Verification items for the finished model (mm, model axes). Face numbers are marked on the shaded views. A direction names the side the tool comes from. Coordinates: 2 decimals unless noted, no trailing zeros. Write each loop counter-clockwise with the first axis right and the second up, starting at its lowest first coordinate (ties: lowest second). Pieces come first, ordered by that corner, then holes. Notation, with made-up numbers: M 54.5,58.5 L 88.5,58.5 A6 ccw 88.5,67.5 Z; hole C 6,-30 d11. An arc over 180 degrees is marked long. Answer in a Markdown table with one row per item.
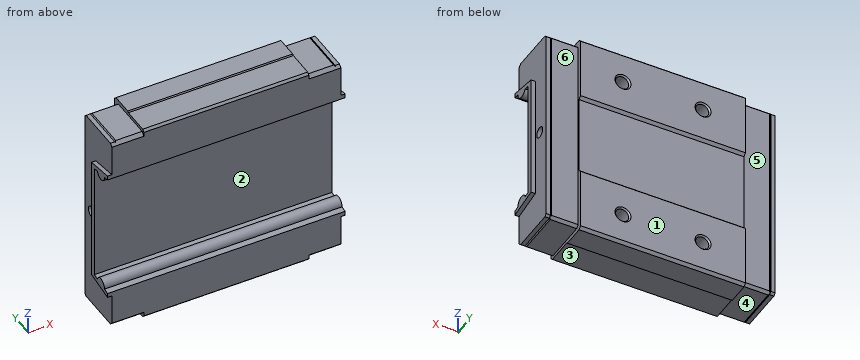
from build123d import *

# Parameters (mm, degrees)
RESSALTO_EXTRUS_O1_DEPTH      = 15.45
RESSALTO_EXTRUS_O1_DEPTH_BACK = 15.45
RESSALTO_EXTRUS_O2_DEPTH      = 6
RESSALTO_EXTRUS_O3_DEPTH      = 6
RESSALTO_EXTRUS_O4_DEPTH      = 22.25
RESSALTO_EXTRUS_O4_DEPTH_BACK = 22.25
CORTE_EXTRUS_O1_DEPTH         = 22.25
CORTE_EXTRUS_O1_DEPTH_BACK    = 22.25
ESBO_O10_W                    = 48.5
ESBO_O10_H                    = 44
CORTE_EXTRUS_O2_DEPTH         = 11
CORTE_EXTRUS_O3_DEPTH         = 20
CORTE_EXTRUS_O3_DEPTH_BACK    = 20
CORTE_EXTRUS_O4_DEPTH         = 20
CORTE_EXTRUS_O4_DEPTH_BACK    = 20
CORTE_EXTRUS_O5_DEPTH         = 10
CORTE_EXTRUS_O6_DEPTH         = 10
CORTE_EXTRUS_O7_DEPTH         = 10
CORTE_EXTRUS_O8_DEPTH         = 10
ESBO_O17_W                    = 2.5
ESBO_O17_H                    = 1
ESBO_O18_W                    = 2.5
ESBO_O18_H                    = 1


with BuildPart() as part:
    # Esboço1 → Ressalto-extrusão1 (new, two sides: drawn at the far end of the back side and taken through both)
    with BuildSketch(Plane(origin=(0, 0, 0), x_dir=(0, 0, -1), z_dir=(1, 0, 0)).offset(-RESSALTO_EXTRUS_O1_DEPTH_BACK)):
        Polygon((-20, 9.5), (-20, 5.5), (-19.8, 5.3), (-19.8, 0.4), (-19.4, 0), (19.4, 0), (19.8, 0.4), (19.8, 5.3), (20, 5.5), (20, 9.5), (19.5, 10), (8, 10), (7.5, 9.5), (-7.5, 9.5), (-8, 10), (-19.5, 10), align=None)
    extrude(amount=RESSALTO_EXTRUS_O1_DEPTH + RESSALTO_EXTRUS_O1_DEPTH_BACK)

    # Esboço2 → Ressalto-extrusão2 (add)
    with BuildSketch(Plane(origin=(-15.45, 0, 0), x_dir=(0, 0, -1), z_dir=(1, 0, 0))):
        Polygon((-19.2, 8.7), (-19.2, 0.6), (-18.6, 0), (18.6, 0), (19.2, 0.6), (19.2, 8.7), (18.7, 9.2), (-18.7, 9.2), align=None)
    extrude(amount=-RESSALTO_EXTRUS_O2_DEPTH)

    # Esboço3 → Ressalto-extrusão3 (add)
    with BuildSketch(Plane(origin=(15.45, 0, 0), x_dir=(0, 0, -1), z_dir=(1, 0, 0))):
        Polygon((-19.2, 8.7), (-19.2, 0.6), (-18.6, 0), (18.6, 0), (19.2, 0.6), (19.2, 8.7), (18.7, 9.2), (-18.7, 9.2), align=None)
    extrude(amount=RESSALTO_EXTRUS_O3_DEPTH)

    # Esboço4 → Ressalto-extrusão4 (add, two sides: drawn at the far end of the back side and taken through both)
    with BuildSketch(Plane(origin=(0, 0, 0), x_dir=(0, 0, -1), z_dir=(1, 0, 0)).offset(-RESSALTO_EXTRUS_O4_DEPTH_BACK)):
        Polygon((-12.816, 0), (12.816, 0), (11.846201606, 5.5), (-11.846201606, 5.5), align=None)
    extrude(amount=RESSALTO_EXTRUS_O4_DEPTH + RESSALTO_EXTRUS_O4_DEPTH_BACK)

    # Esboço5 → Corte-extrusão1 (cut, two sides: drawn at the far end of the back side and taken through both)
    with BuildSketch(Plane(origin=(0, 0, 0), x_dir=(0, 0, -1), z_dir=(1, 0, 0)).offset(-CORTE_EXTRUS_O1_DEPTH_BACK)):
        with BuildLine():
            Line((-12, 0), (12, 0))
            Line((12, 0), (11.814562479, 1.051668439))
            ThreePointArc((11.814562479, 1.051668439), (10.518990309, 2.082939778), (11.383714346, 3.495129625))
            Line((11.383714346, 3.495129625), (11.206528587, 4.5))
            Line((11.206528587, 4.5), (-11.206528587, 4.5))
            Line((-11.206528587, 4.5), (-11.383714346, 3.495129625))
            ThreePointArc((-11.383714346, 3.495129625), (-10.518990309, 2.082939778), (-11.814562479, 1.051668439))
            Line((-11.814562479, 1.051668439), (-12, 0))
        make_face()
    extrude(amount=CORTE_EXTRUS_O1_DEPTH + CORTE_EXTRUS_O1_DEPTH_BACK, mode=Mode.SUBTRACT)

    # Esboço6 → Corte-Revolução1 (revolve, cut)
    with BuildSketch(Plane.XY.offset(14), mode=Mode.PRIVATE) as corte_revolu_o1_sk:
        Polygon((7.5, 10), (9, 10), (8.7295, 9.7295), (8.7295, 5.8), (7.5, 5.090147844), align=None)
    revolve(corte_revolu_o1_sk.sketch.rotate(Axis((7.5, 5.090147844, 14), (0, 1, 0)), 270), axis=Axis((7.5, 5.090147844, 14), (0, 1, 0)), mode=Mode.SUBTRACT)

    # Esboço7 → Corte-Revolução2 (revolve, cut)
    with BuildSketch(Plane.XY.offset(-14), mode=Mode.PRIVATE) as corte_revolu_o2_sk:
        Polygon((-7.5, 10), (-6, 10), (-6.2705, 9.7295), (-6.2705, 5.8), (-7.5, 5.090147844), align=None)
    revolve(corte_revolu_o2_sk.sketch.rotate(Axis((-7.5, 5.090147844, -14), (0, 1, 0)), 270), axis=Axis((-7.5, 5.090147844, -14), (0, 1, 0)), mode=Mode.SUBTRACT)

    # Esboço8 → Corte-Revolução3 (revolve, cut)
    with BuildSketch(Plane.XY.offset(14), mode=Mode.PRIVATE) as corte_revolu_o3_sk:
        Polygon((-7.5, 10), (-6, 10), (-6.2705, 9.7295), (-6.2705, 5.8), (-7.5, 5.090147844), align=None)
    revolve(corte_revolu_o3_sk.sketch.rotate(Axis((-7.5, 5.090147844, 14), (0, 1, 0)), 270), axis=Axis((-7.5, 5.090147844, 14), (0, 1, 0)), mode=Mode.SUBTRACT)

    # Esboço9 → Corte-Revolução4 (revolve, cut)
    with BuildSketch(Plane.XY.offset(-14), mode=Mode.PRIVATE) as corte_revolu_o4_sk:
        Polygon((7.5, 10), (9, 10), (8.7295, 9.7295), (8.7295, 5.8), (7.5, 5.090147844), align=None)
    revolve(corte_revolu_o4_sk.sketch.rotate(Axis((7.5, 5.090147844, -14), (0, 1, 0)), 270), axis=Axis((7.5, 5.090147844, -14), (0, 1, 0)), mode=Mode.SUBTRACT)

    # Esboço10 → Corte-extrusão2 (cut)
    with BuildSketch(Plane(origin=(0, 0, 0), x_dir=(1, 0, 0), z_dir=(0, 1, 0))):
        Rectangle(ESBO_O10_W, ESBO_O10_H)
        Polygon((-23.25, 19.1), (-23.25, -19.1), (-20.65, -19.1), (-20.65, -21), (20.65, -21), (20.65, -19.1), (23.25, -19.1), (23.25, 19.1), (20.65, 19.1), (20.65, 21), (-20.65, 21), (-20.65, 19.1), align=None, mode=Mode.SUBTRACT)
    extrude(amount=CORTE_EXTRUS_O2_DEPTH, mode=Mode.SUBTRACT)

    # Esboço11 → Corte-extrusão3 (cut, two sides: drawn at the far end of the back side and taken through both)
    with BuildSketch(Plane.XY.offset(-CORTE_EXTRUS_O3_DEPTH_BACK)):
        Polygon((-20.65, 9.2), (-20.65, 8.95), (-20.4, 9.2), align=None)
    extrude(amount=CORTE_EXTRUS_O3_DEPTH + CORTE_EXTRUS_O3_DEPTH_BACK, mode=Mode.SUBTRACT)

    # Esboço12 → Corte-extrusão4 (cut, two sides: drawn at the far end of the back side and taken through both)
    with BuildSketch(Plane.XY.offset(-CORTE_EXTRUS_O4_DEPTH_BACK)):
        Polygon((20.4, 9.2), (20.65, 8.95), (20.65, 9.2), align=None)
    extrude(amount=CORTE_EXTRUS_O4_DEPTH + CORTE_EXTRUS_O4_DEPTH_BACK, mode=Mode.SUBTRACT)

    # Esboço13 → Corte-extrusão5 (cut)
    with BuildSketch(Plane(origin=(0, 0, 0), x_dir=(1, 0, 0), z_dir=(0, 1, 0))):
        Polygon((-20.65, 19.2), (-20.65, 18.95), (-20.4, 19.2), align=None)
    extrude(amount=CORTE_EXTRUS_O5_DEPTH, mode=Mode.SUBTRACT)

    # Esboço14 → Corte-extrusão6 (cut)
    with BuildSketch(Plane(origin=(0, 0, 0), x_dir=(1, 0, 0), z_dir=(0, 1, 0))):
        Polygon((-20.65, -19.2), (-20.4, -19.2), (-20.65, -18.95), align=None)
    extrude(amount=CORTE_EXTRUS_O6_DEPTH, mode=Mode.SUBTRACT)

    # Esboço15 → Corte-extrusão7 (cut)
    with BuildSketch(Plane(origin=(0, 0, 0), x_dir=(1, 0, 0), z_dir=(0, 1, 0))):
        Polygon((20.4, 19.2), (20.65, 18.95), (20.65, 19.2), align=None)
    extrude(amount=CORTE_EXTRUS_O7_DEPTH, mode=Mode.SUBTRACT)

    # Esboço16 → Corte-extrusão8 (cut)
    with BuildSketch(Plane(origin=(0, 0, 0), x_dir=(1, 0, 0), z_dir=(0, 1, 0))):
        Polygon((20.4, -19.2), (20.65, -19.2), (20.65, -18.95), align=None)
    extrude(amount=CORTE_EXTRUS_O8_DEPTH, mode=Mode.SUBTRACT)

    # Esboço17 → Corte-Revolução5 (revolve, cut)
    with BuildSketch(Plane.XY, mode=Mode.PRIVATE) as corte_revolu_o5_sk:
        with Locations((-20.2, 7.5)):
            Rectangle(ESBO_O17_W, ESBO_O17_H)
    revolve(corte_revolu_o5_sk.sketch.rotate(Axis((-18.95, 7, 0), (-1, 0, 0)), 270), axis=Axis((-18.95, 7, 0), (-1, 0, 0)), mode=Mode.SUBTRACT)

    # Esboço18 → Corte-Revolução6 (revolve, cut)
    with BuildSketch(Plane.XY, mode=Mode.PRIVATE) as corte_revolu_o6_sk:
        with Locations((20.2, 7.5)):
            Rectangle(ESBO_O18_W, ESBO_O18_H)
    revolve(corte_revolu_o6_sk.sketch.rotate(Axis((21.45, 7, 0), (-1, 0, 0)), 270), axis=Axis((21.45, 7, 0), (-1, 0, 0)), mode=Mode.SUBTRACT)


solid = part.part
1) Tool access check on the marked faces 4, 5 and 6. Record the directions out of +Z, -Z, +X, -X, +Y, -Y that give a thin tool (end or side, any length) a straight path to the whole face; none if there is none.
Response values:
| item | result |
|---|---|
| face 4 | -Z, -X, +Y, -Y |
| face 5 | +Z, -Z, -X, +Y |
| face 6 | +Z, -Z, +X, +Y |
2) Thickness scan on L1, parallel to X at y = 6.65, z = -14; L2, parallel to Z at x = 1, y = 1. Record the ranges inside material, lowest first. Write a range as [from, to].
Response values:
| item | result |
|---|---|
| L1 | x = [-21.45, -8.73], [-6.27, 6.27], [8.73, 21.45] |
| L2 | z = [-19.8, -11.82], [11.82, 19.8] |
3) Release check for a two-part mould opening along Z. For the marked faces 1, 2 and 3 record: +Z half, -Z half, draft (parallel to the pull), parting line (faces both ways), or undercut.
Response values:
| item | result |
|---|---|
| face 1 | draft |
| face 2 | undercut |
| face 3 | -Z half |
4) Depth check by flat-ended pin: pin 1 (1.5 mm diameter, centred on x = -18, y = 4.5, fed in from +Z); pin 2 (1.5 mm diameter, centred on y = 3.5, z = -2.5, fed in from +X); pin 3 (2 mm diameter, centred on x = -2.5, y = 1.5, fed in from +Z); pin 4 (4 mm diameter, centred on x = -17.5, z = -4, fed in from +Y). Enter the tip coordinate at first touch or a pass-through.
Response values:
| item | result |
|---|---|
| pin 1 | stops at z = 19.2 |
| pin 2 | passes through |
| pin 3 | stops at z = 19.8 |
| pin 4 | stops at y = 9.2 |
5) Sectioned sample at D-D (z = 0). Record the cut outline in (x, y), then the cut area to 3 significant figures.
Response values:
| item | result |
|---|---|
| outline | M -22.25,4.5 L 22.25,4.5 L 22.25,5.5 L 21.45,5.5 L 21.45,6 L 18.95,6 L 18.95,8 L 21.45,8 L 21.45,9.2 L 20.65,9.2 L 20.65,8.95 L 20.4,9.2 L 15.45,9.2 L 15.45,9.5 L -15.45,9.5 L -15.45,9.2 L -20.4,9.2 L -20.65,8.95 L -20.65,9.2 L -21.45,9.2 L -21.45,8 L -18.95,8 L -18.95,6 L -21.45,6 L -21.45,5.5 L -22.25,5.5 Z |
| area | 202 mm² |
6) Sectioned sample at A-A (z = -7). Record the cut outline in (x, y).
Response values:
| item | result |
|---|---|
| outline | M -22.25,4.5 L 22.25,4.5 L 22.25,5.5 L 21.45,5.5 L 21.45,9.2 L 20.65,9.2 L 20.65,8.95 L 20.4,9.2 L 15.45,9.2 L 15.45,9.5 L -15.45,9.5 L -15.45,9.2 L -20.4,9.2 L -20.65,8.95 L -20.65,9.2 L -21.45,9.2 L -21.45,5.5 L -22.25,5.5 Z |
7) Sectioned sample at C-C (y = 7). Give the number of separate pieces and of enclosed holes in the cut face, then the cut area to 3 significant figures.
Response values:
| item | result |
|---|---|
| separate pieces | 1 |
| enclosed holes | 4 |
| area | 1,670 mm² |
8) Sectioned sample at B-B (x = 13). Record the cut outline in (y, z), then the cut area to 3 significant figures.
Response values:
| item | result |
|---|---|
| outline | M 0,-19.4 L 0.4,-19.8 L 5.3,-19.8 L 5.5,-20 L 9.5,-20 L 10,-19.5 L 10,-8 L 9.5,-7.5 L 9.5,7.5 L 10,8 L 10,19.5 L 9.5,20 L 5.5,20 L 5.3,19.8 L 0.4,19.8 L 0,19.4 L 0,12 L 1.05,11.81 A1.25 ccw 3.5,11.38 L 4.5,11.21 L 4.5,-11.21 L 3.5,-11.38 A1.25 ccw 1.05,-11.81 L 0,-12 Z |
| area | 289 mm² |
